Input: part model. Units: mm. Frame: model coordinates. Coordinates: 2 decimals unless noted, no trailing zeros. Loops run counter-clockwise (first coordinate to the right, second up) from the corner with the lowest first, then second, coordinate; pieces in that order, holes last.
Item 1: Section A-A on x = 0. Return loops of the section in (y, z).
Item 2: Section B-B on z = -1.5. Return loops of the section in (x, y).
Item 3: Contact query for a flat-ended pin moving along its axis: P1, Ø1.3, axis at x = -0.5, y = -6.5, coming from the -Z side. Output: stop coordinate, or through.
Item 4: Section D-D on z = 1.75. Return loops of the section in (x, y), and give its area (3 significant figures).
Item 5: Section C-C on y = -4. Return loops of the section in (x, z), and give its area (3 significant figures).
Item 6: Ray query, line 1 along Z through (x, y) = (-0.35, -8.5); line 2 along Z through (x, y) = (1.7, -5); line 3 along X through (y, z) = (0.25, 2.25). Return the intervals inside material, ascending.
```python
from build123d import *

# Parameters (mm, degrees)
SKETCH_2_W      = 4.2
SKETCH_2_H      = 13
EXTRUDE_1_DEPTH = 9
SKETCH_3_R      = 0.3
EXTRUDE_2_DEPTH = 4
FILLET_1_R      = 1.5


with BuildPart() as part:
    # Эскиз2 → Бобышка-Вытянуть1 (new body)
    with BuildSketch(Plane.XY):
        with Locations((0, -5)):
            Rectangle(SKETCH_2_W, SKETCH_2_H)
    extrude(amount=EXTRUDE_1_DEPTH)

    # Эскиз3 → Бобышка-Вытянуть2 (add)
    with BuildSketch(Plane(origin=(0, 0, 0), x_dir=(-1, 0, 0), z_dir=(0, 0, -1))):
        Circle(SKETCH_3_R)
        with Locations((0, -10)):
            Circle(SKETCH_3_R)
    extrude(amount=EXTRUDE_2_DEPTH)

    # Скругление1
    fillet_1_edges = [part.edges().sort_by_distance(p)[0] for p in [
        (2.1, -5, 9),
        (0, 1.5, 9),
        (-2.1, -5, 9),
        (0, -11.5, 9),
        (-2.1, 1.5, 4.5),
        (2.1, 1.5, 4.5),
        (2.1, -11.5, 4.5),
        (-2.1, -11.5, 4.5),
    ]]
    fillet(fillet_1_edges, radius=FILLET_1_R)


solid = part.part
```
Results found:
1. outline: (-11.5, 0) - (-10.3, 0) - (-10.3, -4) - (-9.7, -4) - (-9.7, 0) - (-0.3, 0) - (-0.3, -4) - (0.3, -4) - (0.3, 0) - (1.5, 0) - (1.5, 7.5) arc R1.5 ccw to (0, 9) - (-10, 9) arc R1.5 ccw to (-11.5, 7.5) - close
2. outline: circle Ø0.6 at (0, -10); circle Ø0.6 at (0, 0)
3. P1: stops at z = 0
4. outline: (-2.1, -10) arc R1.5 ccw to (-0.6, -11.5) - (0.6, -11.5) arc R1.5 ccw to (2.1, -10) - (2.1, 0) arc R1.5 ccw to (0.6, 1.5) - (-0.6, 1.5) arc R1.5 ccw to (-2.1, 0) - close
4. area: 52.7 mm2
5. outline: (-2.1, 0) - (2.1, 0) - (2.1, 7.5) arc R1.5 ccw to (0.6, 9) - (-0.6, 9) arc R1.5 ccw to (-2.1, 7.5) - close
5. area: 36.8 mm2
6. line 1: z = 0 to 9
6. line 2: z = 0 to 8.52
6. line 3: x = -2.08 to 2.08
